from build123d import *

# Parameters (mm, degrees)
BOSS_EXTRUDE1_DEPTH = 100
SKETCH5_R           = 1.5
CUT_EXTRUDE3_DEPTH  = 4
CUT_EXTRUDE5_REACH  = 130.673
CUT_EXTRUDE6_REACH  = 115.839
SKETCH11_R          = 1.25
CUT_EXTRUDE4_DEPTH  = 2


with BuildPart() as part:
    # Sketch1 → Boss-Extrude1 (new body)
    with BuildSketch(Plane(origin=(0, 0, 0), x_dir=(0, 0, -1), z_dir=(1, 0, 0))):
        Polygon((-25.195982579, -13.090802774), (-33.195982579, -13.090802774), (-33.195982579, 10.909197226), (-29.195982579, 14.909197226), (37.992717903, 14.909197226), (41.992717903, 10.909197226), (41.992717903, -13.090802774), (33.992717903, -13.090802774), (33.992717903, -15.090802774), (43.992717903, -15.090802774), (43.992717903, 11.73762435), (38.821145028, 16.909197226), (-30.024409703, 16.909197226), (-35.195982579, 11.73762435), (-35.195982579, -15.090802774), (-25.195982579, -15.090802774), align=None)
    extrude(amount=BOSS_EXTRUDE1_DEPTH)

    # Sketch5 → Cut-Extrude3 (cut)
    with BuildSketch(Plane.XZ.offset(15.090802774)):
        with Locations(Location((5, 30.195982579, 0), (0, 0, 270))):
            Circle(SKETCH5_R)
        with Locations(Location((92, 30.195982579, 0), (0, 0, 270))):
            Circle(SKETCH5_R)
        with Locations(Location((92, -38.992717903, 0), (0, 0, 270))):
            Circle(SKETCH5_R)
        with Locations(Location((5, -38.992717903, 0), (0, 0, 270))):
            Circle(SKETCH5_R)
    extrude(amount=-CUT_EXTRUDE3_DEPTH, mode=Mode.SUBTRACT)

    # Sketch10 → Cut-Extrude5 (cut, up to next)
    with BuildSketch(Plane.XY.offset(35.195982579), mode=Mode.PRIVATE) as cut_extrude5_sk1:
        with BuildLine():
            Line((11.390334367, 10), (88.31435142, 10))
            ThreePointArc((88.31435142, 10), (91.849885326, 8.535533906), (93.31435142, 5))
            Line((93.31435142, 5), (93.31435142, -5))
            ThreePointArc((93.31435142, -5), (91.849885326, -8.535533906), (88.31435142, -10))
            Line((88.31435142, -10), (11.390334367, -10))
            ThreePointArc((11.390334367, -10), (7.854800461, -8.535533906), (6.390334367, -5))
            Line((6.390334367, -5), (6.390334367, 5))
            ThreePointArc((6.390334367, 5), (7.854800461, 8.535533906), (11.390334367, 10))
        make_face()
    cut_extrude5_tool1 = extrude(cut_extrude5_sk1.sketch, amount=-CUT_EXTRUDE5_REACH, mode=Mode.PRIVATE) & part.part
    add(cut_extrude5_tool1.solids().sort_by_distance((49.852343, 0, 35.195983))[0], mode=Mode.SUBTRACT)

    # Sketch11 → Cut-Extrude6 (cut, up to next)
    with BuildSketch(Plane(origin=(0, 16.909197226, 0), x_dir=(1, 0, 0), z_dir=(0, 1, 0)), mode=Mode.PRIVATE) as cut_extrude6_sk1:
        with Locations(Location((19.971775687, -7.910031108, 0), (0, 0, 270))):
            Circle(SKETCH11_R)
    cut_extrude6_tool1 = extrude(cut_extrude6_sk1.sketch, amount=-CUT_EXTRUDE6_REACH, mode=Mode.PRIVATE) & part.part
    # Sketch11 → Cut-Extrude6 (cut, up to next)
    with BuildSketch(Plane(origin=(0, 16.909197226, 0), x_dir=(1, 0, 0), z_dir=(0, 1, 0)), mode=Mode.PRIVATE) as cut_extrude6_sk2:
        with Locations(Location((91.79572832, -16.355424806, 0), (0, 0, 270))):
            Circle(SKETCH11_R)
    cut_extrude6_tool2 = extrude(cut_extrude6_sk2.sketch, amount=-CUT_EXTRUDE6_REACH, mode=Mode.PRIVATE) & part.part
    # Sketch11 → Cut-Extrude6 (cut, up to next)
    with BuildSketch(Plane(origin=(0, 16.909197226, 0), x_dir=(1, 0, 0), z_dir=(0, 1, 0)), mode=Mode.PRIVATE) as cut_extrude6_sk3:
        with Locations(Location((16.318342756, -1.387534759, 0), (0, 0, 270))):
            Circle(SKETCH11_R)
    cut_extrude6_tool3 = extrude(cut_extrude6_sk3.sketch, amount=-CUT_EXTRUDE6_REACH, mode=Mode.PRIVATE) & part.part
    # Sketch11 → Cut-Extrude6 (cut, up to next)
    with BuildSketch(Plane(origin=(0, 16.909197226, 0), x_dir=(1, 0, 0), z_dir=(0, 1, 0)), mode=Mode.PRIVATE) as cut_extrude6_sk4:
        with Locations(Location((88.142295389, -9.832928457, 0), (0, 0, 270))):
            Circle(SKETCH11_R)
    cut_extrude6_tool4 = extrude(cut_extrude6_sk4.sketch, amount=-CUT_EXTRUDE6_REACH, mode=Mode.PRIVATE) & part.part
    add(cut_extrude6_tool1.solids().sort_by_distance((19.971776, 16.909197, 7.910031))[0], mode=Mode.SUBTRACT)
    add(cut_extrude6_tool2.solids().sort_by_distance((91.795728, 16.909197, 16.355425))[0], mode=Mode.SUBTRACT)
    add(cut_extrude6_tool3.solids().sort_by_distance((16.318343, 16.909197, 1.387535))[0], mode=Mode.SUBTRACT)
    add(cut_extrude6_tool4.solids().sort_by_distance((88.142295, 16.909197, 9.832928))[0], mode=Mode.SUBTRACT)

    # Sketch7 → Cut-Extrude4 (cut)
    with BuildSketch(Plane(origin=(0, 16.909197226, 0), x_dir=(1, 0, 0), z_dir=(0, 1, 0))):
        with BuildLine():
            Line((39.419167918, 6.398367662), (60.580832082, 6.398367662))
            ThreePointArc((60.580832082, 6.398367662), (62.580832082, 4.398367662), (60.580832082, 2.398367662))
            Line((60.580832082, 2.398367662), (39.419167918, 2.398367662))
            ThreePointArc((39.419167918, 2.398367662), (37.419167918, 4.398367662), (39.419167918, 6.398367662))
        make_face()
    extrude(amount=-CUT_EXTRUDE4_DEPTH, mode=Mode.SUBTRACT)


solid = part.part
Design review of the part built by this model. Coordinates are the model's own, in mm. A direction names the side the tool comes from. Give positions to 0.01 mm unless a question says otherwise; leave off trailing zeros. Order: outer loops, then holes, each group sorted by start corner. A loop starts at its lowest first (then second) coordinate and runs counter-clockwise, first axis right, second up.
1. To check wall thickness, follow L1, parallel to Z at x = 87, y = -11; L2, parallel to Y at x = 19, z = 29; L3, parallel to Y at x = 19.5, z = -11. State the ranges of each line that lie inside material, in increasing order.
Solution:
L1: z = -43.99 to -41.99, 33.2 to 35.2
L2: y = -15.09 to -13.09, 14.91 to 16.91
L3: y = 14.91 to 16.91
2. For pin 1 Ø4 at (x, z) = (92, -38.99) entering from +Y; pin 2 Ø2 at (x, z) = (88.14, 9.83) entering from -Y (1 decimal); pin 3 Ø1 at (x, y) = (53.5, 16) entering from -Z; pin 4 Ø6 at (x, z) = (78.5, -4.5) entering from -Y, all flat-tipped, find the tip position at first contact; note any pin that passes through.
Solution:
pin 1: stops at y = 16.91
pin 2: passes through
pin 3: stops at z = -40.23
pin 4: stops at y = 14.91
3. Add section B-B, the plane x = 85.5. State the section outline as (y, z) points.
Solution:
outline: (-15.09, -43.99) - (11.74, -43.99) - (16.91, -38.82) - (16.91, 30.02) - (11.74, 35.2) - (10, 35.2) - (10, 33.2) - (10.91, 33.2) - (14.91, 29.2) - (14.91, -37.99) - (10.91, -41.99) - (-13.09, -41.99) - (-13.09, -33.99) - (-15.09, -33.99) - close; (-15.09, 25.2) - (-13.09, 25.2) - (-13.09, 33.2) - (-10, 33.2) - (-10, 35.2) - (-15.09, 35.2) - close
4. Add section D-D, the plane y = -3. State the section outline as (x, z) points, then the cut area to 3 significant figures.
Solution:
outline: (0, -43.99) - (100, -43.99) - (100, -41.99) - (0, -41.99) - close; (0, 33.2) - (6.39, 33.2) - (6.39, 35.2) - (0, 35.2) - close; (93.31, 33.2) - (100, 33.2) - (100, 35.2) - (93.31, 35.2) - close
area: 226 mm2
5. Tool access review of faces 1 (the flat face through (50, -11, 33.196)), 2 (the cylindrical face through (5.451, -14.105, -40.423)), 3 (the cylindrical face through (7.82, 8.5, 34.21)), 4 (the flat face through (49, -14, 25.196)): name each direction out of +Z, -Z, +X, -X, +Y, -Y from which nothing blocks a thin tool from reaching the whole face with its end or side.
Solution:
face 1: +X, -X
face 2: -Y
face 3: +Z
face 4: +X, -X, -Y
6. Add section C-C, the plane x = 5. State the section outline as (y, z) points.
Solution:
outline: (-15.09, -43.99) - (11.74, -43.99) - (16.91, -38.82) - (16.91, 30.02) - (11.74, 35.2) - (-15.09, 35.2) - (-15.09, 31.7) - (-13.09, 31.7) - (-13.09, 33.2) - (10.91, 33.2) - (14.91, 29.2) - (14.91, -37.99) - (10.91, -41.99) - (-13.09, -41.99) - (-13.09, -40.49) - (-15.09, -40.49) - close; (-15.09, -37.49) - (-13.09, -37.49) - (-13.09, -33.99) - (-15.09, -33.99) - close; (-15.09, 25.2) - (-13.09, 25.2) - (-13.09, 28.7) - (-15.09, 28.7) - close
7. Add section A-A, the plane y = -12. State the section outline as (x, z) points.
Solution:
outline: (0, -43.99) - (100, -43.99) - (100, -41.99) - (0, -41.99) - close; (0, 33.2) - (100, 33.2) - (100, 35.2) - (0, 35.2) - close
8. Mouldability with a two-part tool opening along Z and no side actions: class faces 5 (the flat face through (49.3, 14.29, -41.44)), 6 (the cylindrical face through (87.033, 15.923, 10.41)), 7 (the flat face through (49, -15.091, -39)) as +Z half, -Z half, draft (parallel to the pull), parting line (faces both ways), or undercut.
Solution:
face 5: -Z half
face 6: undercut
face 7: draft
